Check sheet for the modelled part. Datum: model origin and axes. Units: mm. A direction names the side the tool comes from. Give positions to 0.01 mm unless a question says otherwise; leave off trailing zeros. Order: outer loops, then holes, each group sorted by start corner. A loop starts at its lowest first (then second) coordinate and runs counter-clockwise, first axis right, second up. Notation, with made-up numbers: M 75,-19.5 L 108,-19.5 A19 cw 108,-14.5 Z; hole C -23.75,-2 d2. An arc over 180 degrees is marked long. Answer in a Markdown table with one row per item. Add a question column.
from build123d import *

# Parameters (mm, degrees)
BOSS_EXTRUDE1_DEPTH  = 2
SKETCH3_W            = 21.7
SKETCH3_H            = 0.5
BOSS_EXTRUDE2_DEPTH  = 2
SKETCH2_W            = 2
SKETCH2_H            = 3
CUT_EXTRUDE1_DEPTH   = 2
CHAMFER1_SIZE        = 2
CHAMFER3_SIZE        = 2
BOSS_EXTRUDE3_DEPTH  = 2
SKETCH5_W            = 2
SKETCH5_H            = 3
CUT_EXTRUDE2_DEPTH   = 10
SKETCH8_W            = 0.75
SKETCH8_H            = 10.6
CUT_EXTRUDE5_DEPTH   = 41.850764987
FILLET2_R            = 1
FILLET3_R            = 3
FILLET4_R            = 3
CUT_EXTRUDE4_START   = 30.85
CUT_EXTRUDE4_DEPTH   = 0.8
CUT_EXTRUDE4_START_2 = 0.05
CUT_EXTRUDE4_2_DEPTH = 0.8


# Read off the part's stored shape, not the designer's step: Cut-Extrude4
with BuildPart() as part:
    # Sketch1 → Boss-Extrude1 (new body)
    with BuildSketch(Plane.XY):
        with BuildLine():
            ThreePointArc((2.05, 7.55), (3.55, 9.05), (2.05, 10.55))
            Line((2.05, 10.55), (0.05, 10.55))
            Line((0.05, 10.55), (0.05, 31.65))
            Line((0.05, 31.65), (25.75, 31.65))
            Line((25.75, 31.65), (25.75, 0.05))
            Line((25.75, 0.05), (18.9, 0.05))
            Line((18.9, 0.05), (18.9, 6.05))
            Line((18.9, 6.05), (6.9, 6.05))
            Line((6.9, 6.05), (6.9, 0.05))
            Line((6.9, 0.05), (0.05, 0.05))
            Line((0.05, 0.05), (0.05, 7.55))
            Line((0.05, 7.55), (2.05, 7.55))
        make_face()
        with BuildLine():
            Line((2.05, 2.55), (2.05, 6.3))
            ThreePointArc((2.05, 6.3), (4.8, 9.05), (2.05, 11.8))
            Line((2.05, 11.8), (2.05, 29.65))
            Line((2.05, 29.65), (23.75, 29.65))
            Line((23.75, 29.65), (23.75, 2.55))
            Line((23.75, 2.55), (20.9, 2.55))
            Line((20.9, 2.55), (20.9, 8.05))
            Line((20.9, 8.05), (4.9, 8.05))
            Line((4.9, 8.05), (4.9, 2.55))
            Line((4.9, 2.55), (2.05, 2.55))
        make_face(mode=Mode.SUBTRACT)
    boss_extrude1 = extrude(amount=BOSS_EXTRUDE1_DEPTH)

    # Mirror8: Boss-Extrude1 across plane
    add(boss_extrude1.mirror(Plane.ZY.offset(-12.9)))

    # Sketch3 → Boss-Extrude2 (add)
    with BuildSketch(Plane.XY.offset(2)):
        with Locations((12.9, 29.4)):
            Rectangle(SKETCH3_W, SKETCH3_H)
    extrude(amount=-BOSS_EXTRUDE2_DEPTH)

    # Sketch2 → Cut-Extrude1 (cut)
    with BuildSketch(Plane.XY.offset(2)):
        with Locations((1.05, 9.05)):
            Rectangle(SKETCH2_W, SKETCH2_H)
        with Locations((24.75, 9.05)):
            Rectangle(SKETCH2_W, SKETCH2_H)
    extrude(amount=-CUT_EXTRUDE1_DEPTH, mode=Mode.SUBTRACT)

    # Chamfer1
    chamfer1_edges = [part.edges().sort_by_distance(p)[0] for p in [
        (22.325, 0.05, 2),
        (3.475, 0.05, 2),
    ]]
    chamfer(chamfer1_edges, length=CHAMFER1_SIZE - 0.0001)  # a hair under: the kernel refuses the full size

    # Chamfer3
    chamfer3_edges = [part.edges().sort_by_distance(p)[0] for p in [
        (12.9, 31.65, 2),
    ]]
    chamfer(chamfer3_edges, length=CHAMFER3_SIZE - 0.0001)  # a hair under: the kernel refuses the full size

    # Sketch4 → Boss-Extrude3 (add)
    with BuildSketch(Plane.XY.offset(2)):
        with BuildLine():
            ThreePointArc((2.05, 19.9), (4.8, 22.65), (2.05, 25.4))
            Line((2.05, 25.4), (2.05, 24.15))
            ThreePointArc((2.05, 24.15), (3.55, 22.65), (2.05, 21.15))
            Line((2.05, 21.15), (2.05, 19.9))
        make_face()
        with BuildLine():
            Line((23.75, 24.15), (23.75, 25.4))
            ThreePointArc((23.75, 25.4), (21, 22.65), (23.75, 19.9))
            Line((23.75, 19.9), (23.75, 21.15))
            ThreePointArc((23.75, 21.15), (22.25, 22.65), (23.75, 24.15))
        make_face()
    extrude(amount=-BOSS_EXTRUDE3_DEPTH)

    # Sketch5 → Cut-Extrude2 (cut)
    with BuildSketch(Plane.XY.offset(2)):
        with Locations((1.05, 22.65)):
            Rectangle(SKETCH5_W, SKETCH5_H)
        with Locations((24.75, 22.65)):
            Rectangle(SKETCH5_W, SKETCH5_H)
    extrude(amount=-CUT_EXTRUDE2_DEPTH, mode=Mode.SUBTRACT)

    # Sketch8 → Cut-Extrude5 (cut, through all)
    with BuildSketch(Plane.XY.offset(2)):
        with Locations((25.375, 15.85)):
            Rectangle(SKETCH8_W, SKETCH8_H)
        with Locations((0.425, 15.85)):
            Rectangle(SKETCH8_W, SKETCH8_H)
    extrude(amount=-CUT_EXTRUDE5_DEPTH, mode=Mode.SUBTRACT)

    # Fillet2
    fillet2_edges = [part.edges().sort_by_distance(p)[0] for p in [
        (2.05, 29.15, 1),
        (23.75, 29.15, 1),
        (2.05, 2.55, 1),
        (4.9, 2.55, 1),
        (20.9, 2.55, 1),
        (23.75, 2.55, 1),
        (18.9, 6.05, 1),
        (6.9, 6.05, 1),
    ]]
    fillet(fillet2_edges, radius=FILLET2_R)

    # Fillet3
    fillet3_edges = [part.edges().sort_by_distance(p)[0] for p in [
        (23.75, 6.3, 1),
        (23.75, 11.8, 1),
        (25.75, 7.55, 1),
        (23.75, 25.4, 1),
        (23.75, 19.9, 1),
        (25.75, 24.15, 1),
        (2.05, 11.8, 1),
        (2.05, 6.3, 1),
        (0.05, 7.55, 1),
        (2.05, 19.9, 1),
        (2.05, 25.4, 1),
        (0.05, 24.15, 1),
        (0.8, 10.55, 1),
        (0.8, 21.15, 1),
        (25, 21.15, 1),
        (25, 10.55, 1),
    ]]
    fillet(fillet3_edges, radius=FILLET3_R)

    # Fillet4
    fillet4_edges = [part.edges().sort_by_distance(p)[0] for p in [
        (4.9, 8.05, 1),
        (20.9, 8.05, 1),
    ]]
    fillet(fillet4_edges, radius=FILLET4_R)

    # Cut-Extrude4 outline → Cut-Extrude4 (cut)
    with BuildSketch(Plane(origin=(0, 0, 0), x_dir=(1, 0, 0), z_dir=(0, 1, 0)).offset(CUT_EXTRUDE4_START)):
        Polygon((-1, 1), (-1, -2), (0.05, -2), (25.75, -2), (27, -2), (27, 1), align=None)
    extrude(amount=CUT_EXTRUDE4_DEPTH, mode=Mode.SUBTRACT)

    # Cut-Extrude4 2 outline → Cut-Extrude4 2 (cut)
    with BuildSketch(Plane(origin=(0, 0, 0), x_dir=(1, 0, 0), z_dir=(0, 1, 0)).offset(CUT_EXTRUDE4_START_2)):
        Polygon((6.9, -2), (6.9, 1), (-1, 1), (-1, -2), (0.05, -2), align=None)
        Polygon((18.9, 1), (18.9, -2), (25.75, -2), (27, -2), (27, 1), align=None)
    extrude(amount=CUT_EXTRUDE4_2_DEPTH, mode=Mode.SUBTRACT)


solid = part.part
Q1. Go/stop test with a flat-tipped pin: pin 1 (0.6 mm diameter, centred on x = 12, z = 1, fed in from -Y). Record where the tip stops, or that it passes through.
Q2. Tool access check on faces 4 (the cylindrical face through (2.42, 26.11, 0.99)), 5 (the cylindrical face through (7.201, 5.765, 1.014)), 6 (the flat face through (25.75, 29, 1)). Record the directions out of +Z, -Z, +X, -X, +Y, -Y that give a thin tool (end or side, any length) a straight path to the whole face; none if there is none.
Q3. Thickness scan on probe 1 along Y at (x, z) = (10.5, 0.75); probe 2 along X at (y, z) = (14.5, 1.3); probe 3 along X at (y, z) = (4, 1.55). Record the ranges inside material, lowest first.
Q4. Cross-section at B-B (x = 20). Record the boundary of the cut face in (y, z), and give its area (3 significant figures).
Q5. Cross-section at C-C (x = 24.25). State how many separate pieces and enclosed holes the cut face has, and give its area (3 significant figures).
Q6. Draft check along Y on faces 1 (the flat face through (6.9, 3, 1)), 2 (the cylindrical face through (4.599, 2.835, 1.014)), 3 (the flat face through (22.3, 0.85, 0.4)). Enter one of: pulls with the +Y half, pulls with the -Y half, needs draft (parallel to the pull), parting line crosses it, or undercut.
Q7. Cross-section at A-A (x = 14.75). Record the boundary of the cut face in (y, z).
Values follow:
| question | item | result |
|---|---|---|
| 1 | pin 1 | y = 6.05 |
| 2 | face 4 | +Z, -Z |
| 2 | face 5 | +Z, -Z, -Y |
| 2 | face 6 | +Z, -Z, +X, +Y, -Y |
| 3 | probe 1 | 6.05 to 8.05, 29.15 to 30.85 |
| 3 | probe 2 | 0.8 to 2.05, 23.75 to 25 |
| 3 | probe 3 | 0.05 to 2.05, 4.9 to 6.9, 18.9 to 20.9, 23.75 to 25.75 |
| 4 | outline | M 0.85,0 L 7.19,0 L 7.19,2 L 2.05,2 L 0.85,0.8 Z; M 29.15,0 L 30.85,0 L 30.85,0.8 L 29.65,2 L 29.15,2 Z |
| 4 | area | 14.6 mm² |
| 5 | separate pieces | 3 |
| 5 | enclosed holes | 0 |
| 5 | area | 42.8 mm² |
| 6 | face 1 | needs draft |
| 6 | face 2 | undercut |
| 6 | face 3 | pulls with the -Y half |
| 7 | outline | M 6.05,0 L 8.05,0 L 8.05,2 L 6.05,2 Z; M 29.15,0 L 30.85,0 L 30.85,0.8 L 29.65,2 L 29.15,2 Z |
